Autodesk Inventor part; units mm, degrees
ref_plane "YZ Plane" through (0, 0, 0) normal (1, 0, 0) x (0, 1, 0)
ref_plane "XZ Plane" through (0, 0, 0) normal (0, 1, 0) x (-1, 0, 0)
ref_plane "XY Plane" through (0, 0, 0) normal (0, 0, 1) x (1, 0, 0)
sketch "Sketch1" plane through (0, 0, 0) normal (0, 0, 1) x (1, 0, 0)
  line L0 (0, 226.8926) -> (200, 226.8926)
  line L1 (200, 226.8926) -> (200, -273.1074)
  line L2 (200, -273.1074) -> (70.0106, -273.1074)
  spline S0 degree 4 poles (0, 177.3413) (126.203, 79.0594) (154.2664, -10.2822) (176.0066, -260.8084) (70.0106, -273.1074) knots 0 0 0 0 0 1 1 1 1 1
  spline S1 degree 2 poles (0, 177.3413) (-36.5043, 204.7595) (-58.7785, 226.8926) knots 0 0 0 1 1 1
  line L3 (-58.7785, 226.8926) -> (0, 226.8926)
  point P0 (0, 0)
  point P1 (99.9997, 63.7426)
  point P2 (140.6791, -78.917)
  point P3 (126.8096, -220.2554)
  point P4 (-35.664, 205.7436)
extrude "Extrusion1" add sketch "Sketch1" along normal blind 10
sketch "Sketch2" plane through (0, 0, 10) normal (0, 0, 1) x (1, 0, 0)
  circle A0 centre (66.8612, 154.6625) radius 5
  circle A1 centre (180.0109, 154.6625) radius 5
  circle A2 centre (185.0109, 38.5738) radius 5
  circle A3 centre (126.375, 38.5738) radius 5
  point P0 (0, 0)
  dimension "d5" = 10
  dimension "d6" = 10
  dimension "d7" = 10
  dimension "d8" = 10
extrude "Extrusion2" add sketch "Sketch2" along normal blind 20
sketch "Sketch3" plane through (180.0109, 154.6625, 30) normal (0, 0, 1) x (1, 0, 0)
  circle A0 centre (-113.1497, 0) radius 5
  circle A1 centre (0, 0) radius 5
  line L0 (-113.1497, 0) -> (0, 0)
  circle A2 centre (5, -116.0887) radius 5
  line L1 (0, 0) -> (5, -116.0887)
  circle A3 centre (-53.6359, -116.0887) radius 5
  line L2 (5, -116.0887) -> (-53.6359, -116.0887)
  spline S0 degree 2 poles (-113.1497, 0) (-63.3738, -35.791) (-53.6359, -116.0887) knots 0 0 0 1 1 1
  point P0 (-180.0109, -154.6625)
  point P1 (-75.6781, -42.6148)
extrude "Extrusion3" add sketch "Sketch3" along normal blind 10 contours L0 A1 L1 A2 L2 A3 S0 A0 | A0 S0 L0 | L0 L1 A1 | A3 L2 S0 | L1 L2 A2 picked at (-110.3004, -1.6927) picked at (-1.6834, -2.8514) picked at (-53.6623, -112.78) picked at (1.7062, -115.7278)
sketch "Sketch4" plane through (180.0109, 154.6625, 40) normal (0, 0, 1) x (1, 0, 0)
  line L0 (-72.7391, -18.3685) -> (-12.7391, -18.3685)
  line L1 (-12.7391, -18.3685) -> (-6.5901, -92.1125)
  spline S0 degree 2 poles (-72.7391, -18.3685) (-51.5746, -50.5042) (-42.859, -93.2077) knots 0 0 0 1 1 1
  line L2 (-14.6388, -92.7837) -> (-19.9394, -29.2142)
  line L3 (-19.9394, -29.2142) -> (-55.1054, -29.2142)
  spline S1 degree 2 poles (-55.1054, -29.2142) (-38.2895, -49.2242) (-32.7381, -93.2077) knots 0 0 0 1 1 1
  line L4 (-42.859, -93.2077) -> (-32.7381, -93.2077)
  line L5 (-14.6388, -92.7837) -> (-6.5901, -92.1125)
  point P0 (-180.0109, -154.6625)
  point P1 (-55.1635, -51.9626)
  point P2 (-42.687, -50.9557)
  dimension "d13" = 60
  dimension "d14" = 74
extrude "Extrusion4" cut sketch "Sketch4" against normal blind 10
sketch "Sketch6" plane through (0, 0, 10) normal (0, 0, 1) x (1, 0, 0)
  line L0 (135.0053, -253.8522) -> (165.0053, -253.8522)
  line L1 (165.0053, -253.8522) -> (165.0053, -260.8522)
  line L2 (165.0053, -260.8522) -> (135.0053, -260.8522)
  line L3 (135.0053, -260.8522) -> (135.0053, -253.8522)
  line L4 (141.0698, -234.749) -> (171.0698, -234.749)
  line L5 (171.0698, -234.749) -> (171.0698, -241.749)
  line L6 (171.0698, -241.749) -> (141.0698, -241.749)
  line L7 (141.0698, -241.749) -> (141.0698, -234.749)
  point P0 (0, 0)
  dimension "d22" = 30
  dimension "d23" = 7
  dimension "d24" = 30
  dimension "d25" = 7
extrude "Extrusion6" add sketch "Sketch6" along normal blind 10
sketch "Sketch8" plane through (0, 0, 0) normal (0, 0, -1) x (-1, 0, 0)
  circle A0 centre (-180.0109, 154.6625) radius 5
  circle A1 centre (-180.0109, 154.6625) radius 5
  line L0 (-180.0109, 154.6625) -> (-154.3956, -221.4322) construction
  circle A2 centre (-154.3956, -221.4322) radius 5
  point P0 (0, 0)
  dimension "d32" = 10
  dimension "d33" = 376.966
  dimension "d34" = 10
extrude "Extrusion8" add sketch "Sketch8" along normal blind 10
properties part number "Part2 new side frame" material "CFRP"
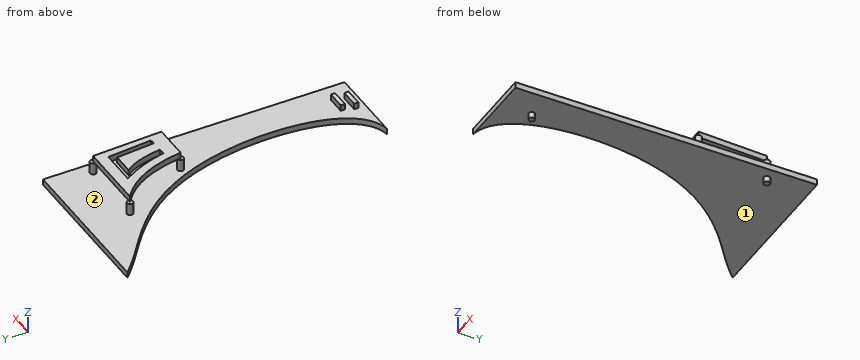
Here's how the part is built. I have some questions about the finished solid (model axes, mm). Face numbers are marked on the shaded views. Coordinates: 2 decimals unless noted, no trailing zeros. Answer as CSV lines item,"result".
Item 1: Imagine slicing it at A-A on x = 78. Give the number of separate pieces and of enclosed holes in the cut face, plus the area to 3 significant figures.
Results found:
separate pieces,"3"
enclosed holes,"0"
area,"1,380 mm2"
Item 2: We'd pull the mould along Z, two halves only. Please class the marked faces 1 and 2: +Z half, -Z half, draft (parallel to the pull), parting line (faces both ways), or undercut.
Results found:
face 1,"-Z half"
face 2,"undercut"
Item 3: If I drill on line 1 (Y direction, x = 126.5, z = 27); line 2 (Z direction, x = 48.5, y = 159); line 3 (Y direction, x = 183.5, z = 28), over which ranges is the centre line in solid material (lowest first)?
Results found:
line 1,"33.58 to 43.57"
line 2,"0 to 10"
line 3,"33.81 to 43.34, 151.08 to 158.24"
Item 4: For pin 1 (1.5 mm diameter, centred on x = 161, y = -27, fed in from +Z); pin 2 (8 mm diameter, centred on x = 142.5, z = 34, fed in from +Y); pin 3 (5.5 mm diameter, centred on y = -256, z = 16, fed in from -X), each with a flat end and sliding along its axis, tell me the tip position at first contact or that it passes through.
Results found:
pin 1,"z = 10"
pin 2,"y = 154.66"
pin 3,"x = 135.01"
